from build123d import *

# Parameters (mm, degrees)
SKETCH_1_R      = 1.5875
EXTRUDE_1_DEPTH = 18


with BuildPart() as part:
    # 草图1 → 凸台-拉伸1 (new body)
    with BuildSketch(Plane(origin=(0, 0, 0), x_dir=(1, 0, 0), z_dir=(0, 1, 0))):
        Polygon((31.8, 26.65), (-34.3, 26.65), (-34.3, -26.65), (34.3, -26.65), (34.3, 13.519706399), (31.8, 16.019706399), align=None)
        with Locations(Location((-20.3, -24.15, 0), (0, 0, 270))):
            Circle(SKETCH_1_R, mode=Mode.SUBTRACT)
        with Locations(Location((31.8, -19.05, 0), (0, 0, 270))):
            Circle(SKETCH_1_R, mode=Mode.SUBTRACT)
        with Locations(Location((-19, 24.05, 0), (0, 0, 270))):
            Circle(SKETCH_1_R, mode=Mode.SUBTRACT)
        with Locations(Location((31.8, 8.85, 0), (0, 0, 270))):
            Circle(SKETCH_1_R, mode=Mode.SUBTRACT)
    extrude(amount=EXTRUDE_1_DEPTH)


solid = part.part
Work out the finished part from the listing and answer in its coordinate system (mm). A direction names the side the tool comes from. Coordinates: 2 decimals unless noted, no trailing zeros. Loops run counter-clockwise (first coordinate to the right, second up) from the corner with the lowest first, then second, coordinate; pieces in that order, holes last. Notation, with made-up numbers: M 51,-32.5 L 70,-32.5 A13 cw 70,-15.5 Z; hole C 63,11.5 d8. An arc over 180 degrees is marked long. Answer in a Markdown table with one row per item. Add a question column.
1. Find section C-C, the plane z = -9.5. Write down the section's boundary in (x, y).
2. Find section A-A, the plane z = 19.05. Write down the section's boundary in (x, y).
3. Find section B-B, the plane y = 1.5. State how many separate pieces and enclosed holes the cut face has, then the cut area to 4 significant figures.
4. A flat-ended cylindrical pin translates along its axis: P1, Ø3, axis at y = 4.5, z = -23.5, coming from the +X side. Find the tip coordinate at first contact, or state that the pin passes through.
5. The mould has two halves that part along Z. Classify faces 3 (the flat face through (0, 9, 26.65)), 4 (the flat face through (-34.3, 9, 0)), 5 (the cylindrical face through (32.873, 8.874, -10.02)): pulls with the +Z half, pulls with the -Z half, needs draft (parallel to the pull), parting line crosses it, or undercut.
6. A tool of negligible diameter and unlimited length cuts with its end or side. For faces 1 (the cylindrical face through (-20.55, 8.87, -24.39)), 2 (the flat face through (31.8, 9, -21)), from which of +Z, -Z, +X, -X, +Y, -Y can it reach the whole face along a straight path? Write none if from no direction.
7. Find section D-D, the plane z = -18. Write down the section's boundary in (x, y).
8. Consider L1, parallel to X at y = 13.25, z = -24.05; L2, parallel to Z at x = -20, y = 3.25; L3, parallel to Z at x = 30.5, y = 8. Determine where each line is inside the solid, lowest interval first.
Reported:
| question | item | result |
|---|---|---|
| 1 | outline | M -34.3,0 L 30.35,0 L 30.35,18 L -34.3,18 Z; M 33.25,0 L 34.3,0 L 34.3,18 L 33.25,18 Z |
| 2 | outline | M -34.3,0 L 30.21,0 L 30.21,18 L -34.3,18 Z; M 33.39,0 L 34.3,0 L 34.3,18 L 33.39,18 Z |
| 3 | separate pieces | 1 |
| 3 | enclosed holes | 4 |
| 3 | area | 3,595 mm^2 |
| 4 | P1 | stops at x = 31.8 |
| 5 | face 3 | pulls with the +Z half |
| 5 | face 4 | needs draft |
| 5 | face 5 | undercut |
| 6 | face 1 | +Y, -Y |
| 6 | face 2 | -Z, +X, +Y, -Y |
| 7 | outline | M -34.3,0 L 31.8,0 L 31.8,18 L -34.3,18 Z |
| 8 | L1 | x = -34.3 to -20.59, -17.41 to 31.8 |
| 8 | L2 | z = -26.65 to -25.28, -22.82 to 22.59, 25.71 to 26.65 |
| 8 | L3 | z = -26.65 to -9.76, -7.94 to 18.14, 19.96 to 26.65 |
